Here's how the part is built. I have some questions about the finished solid (model axes, mm). A direction names the side the tool comes from. Round coordinates to 2 decimals unless told otherwise and drop trailing zeros. Write each loop counter-clockwise with the first axis right and the second up, starting at its lowest first coordinate (ties: lowest second). Pieces come first, ordered by that corner, then holes. Notation, with made-up numbers: (-27, 24.5) - (32, 24.5) arc R26 cw to (32, 62.5) - close; hole circle Ø11 at (74, 38). An arc over 180 degrees is marked (long way). One line per item, written item: value. Start each with the question number.
Item 1: Imagine slicing it at B-B, the plane y = 12.25. Please give me the cut outline in (x, z).
Item 2: If I drill on line 1 (X direction, y = 5.5, z = 0); line 2 (X direction, y = 4.25, z = -1.5); line 3 (Y direction, x = -0.5, z = 2), over which ranges is the centre line in solid material (lowest first)?
Item 3: For P1, Ø1.5, axis at x = 1.5, y = 5, coming from the +Z side; P2, Ø4, axis at x = 0, z = 0, coming from the -Y side; P3, Ø1, axis at x = 4, y = 1.5, coming from the +Z side, each with a flat end and sliding along its axis, tell me the tip position at first contact or that it passes through.
Item 4: Thinking about a two-plate mould opening in Z: for faces 1 (the face through (0.013, 0.106, -5.184)), 2 (the face through (0.77, 6.34, -2.43)), 3 (the face through (-4.5, 0.11, 2.58)), which applies, released by +Z, released by -Z, zero draft, split by the parting line, or undercut?
Item 5: Imagine slicing it at A-A, the plane y = 5.5. Please give me the cut outline in (x, z), then the cut area to 3 significant figures.
Item 6: For faces 4 (the face through (-5, 6, 0)), 5 (the face through (0, 12.5, 0)), which set-ups out of +Z, -Z, +X, -X, +Y, -Y let a thin tool reach every point of the face, with its end or its side?
```python
from build123d import *

# Parameters (mm, degrees)
VYSUNOUT1_DEPTH          = 13.5
SKICA4_R                 = 2.55
ODEBRAT_VYSUNUT_M1_DEPTH = 12.5
ZKOSIT1_SIZE             = 0.6
ZKOSIT1_SIZE2            = 0.346410162


with BuildPart() as part:
    # Skica1 → Vysunout1 (new body)
    with BuildSketch(Plane(origin=(0, 0, 0), x_dir=(1, 0, 0), z_dir=(0, 1, 0))):
        Polygon((5, -2.886751346), (5, 2.886751346), (0, 5.773502692), (-5, 2.886751346), (-5, -2.886751346), (0, -5.773502692), align=None)
    extrude(amount=VYSUNOUT1_DEPTH)

    # Skica2 → Odebrat otočením1 (revolve, cut)
    with BuildSketch(Plane(origin=(0, 0, 0), x_dir=(0, 0, -1), z_dir=(1, 0, 0)), mode=Mode.PRIVATE) as odebrat_oto_en_m1_sk:
        Polygon((-5.773502692, 13.5), (-5.773502692, 10.726497308), (-3, 13.5), align=None)
    revolve(odebrat_oto_en_m1_sk.sketch.rotate(Axis((0, 13.5, 0), (0, -1, 0)), 180), axis=Axis((0, 13.5, 0), (0, -1, 0)), mode=Mode.SUBTRACT)

    # Skica3 → Odebrat otočením2 (revolve, cut)
    with BuildSketch(Plane.XY):
        Polygon((5, 0), (28.382685902, 0), (28.382685902, 13.5), align=None)
    revolve(axis=Axis((0, 0, 0), (0, 1, 0)), mode=Mode.SUBTRACT)

    # Skica4 → Odebrat vysunutím1 (cut)
    with BuildSketch(Plane.XZ):
        with Locations(Location((0, 0, 0), (0, 0, 270))):
            Circle(SKICA4_R)
    extrude(amount=-ODEBRAT_VYSUNUT_M1_DEPTH, mode=Mode.SUBTRACT)

    # Zkosit1
    zkosit1_edges = [part.edges().sort_by_distance(p)[0] for p in [
        (0, 0, 2.55),
    ]]
    zkosit1_side = [part.faces().sort_by_distance(p)[0] for p in [
        (4.207652534, 0, 2.429289317),
    ]]
    chamfer(zkosit1_edges, length=ZKOSIT1_SIZE, length2=ZKOSIT1_SIZE2, reference=zkosit1_side[0])


solid = part.part
```
Values follow:
1. outline: circle Ø8.5 at (0, 0); hole circle Ø5.1 at (0, 0)
2. line 1: x = -5 to -2.55, 2.55 to 5
2. line 2: x = -5 to -2.06, 2.06 to 5
2. line 3: y = 12.5 to 13.5
3. P1: stops at z = 5.34
3. P2: stops at y = 12.5
3. P3: stops at z = 3.75
4. face 1: released by -Z
4. face 2: undercut
4. face 3: released by +Z
5. outline: (-5, -2.89) - (0, -5.77) - (5, -2.89) - (5, 2.89) - (0, 5.77) - (-5, 2.89) - close; hole circle Ø5.1 at (0, 0)
5. area: 66.2 mm^2
6. face 4: +Z, -Z, -X, +Y, -Y
6. face 5: -Y
